The model under review builds one solid part; all positions refer to its coordinate system, in mm. Coordinates: 2 decimals unless noted, no trailing zeros. Write each loop counter-clockwise with the first axis right and the second up, starting at its lowest first coordinate (ties: lowest second). Pieces come first, ordered by that corner, then holes.
1) For line 1 (Y direction, x = 83, z = 0.85); line 2 (X direction, y = 2.5, z = 0.4); line 3 (Y direction, x = -20, z = 0.55), list the stretches that pass through material, from the lowest coordinate up.
2) Add section A-A, the plane x = 0. State the section outline as (y, z) points.
3) Add section C-C, the plane z = 1.5. Give the number of separate pieces and of enclosed holes in the cut face, then the cut area to 3 significant figures.
4) Add section B-B, the plane x = -83. State the section outline as (y, z) points, then the cut area to 3 significant figures.
from build123d import *

# Parameters (mm, degrees)
SKETCH_1_W          = 178
SKETCH_1_H          = 65
EXTRUDE_1_DEPTH     = 3
FILLET_1_R          = 3
SKETCH_2_R          = 2.1
SKETCH_2_R_2        = 12.5
SKETCH_2_R_3        = 11
SKETCH_2_R_4        = 1.8
CUT_EXTRUDE_1_DEPTH = 10


with BuildPart() as part:
    # 草图1 → 凸台-拉伸1 (new body)
    with BuildSketch(Plane.XY):
        Rectangle(SKETCH_1_W, SKETCH_1_H)
    extrude(amount=EXTRUDE_1_DEPTH)

    # 圆角1
    fillet_1_edges = [part.edges().sort_by_distance(p)[0] for p in [
        (-89, 32.5, 1.5),
        (89, 32.5, 1.5),
        (89, -32.5, 1.5),
        (-89, -32.5, 1.5),
    ]]
    fillet(fillet_1_edges, radius=FILLET_1_R)

    # 草图2 → 切除-拉伸1 (cut)
    # profile 1 of 14: a face of its own
    with BuildSketch(Plane.XY.offset(3)):
        with Locations((-83, 27)):
            Circle(SKETCH_2_R)
    # profile 2 of 14: a face of its own
    with BuildSketch(Plane.XY.offset(3)):
        with Locations((-83, 0)):
            Circle(SKETCH_2_R)
    # profile 3 of 14: a face of its own
    with BuildSketch(Plane.XY.offset(3)):
        with Locations((-83, -27)):
            Circle(SKETCH_2_R)
    # profile 4 of 14: a face of its own
    with BuildSketch(Plane.XY.offset(3)):
        Circle(SKETCH_2_R_2)
        Circle(SKETCH_2_R_3, mode=Mode.SUBTRACT)
    # profile 5 of 14: a face of its own
    with BuildSketch(Plane.XY.offset(3)):
        Circle(SKETCH_2_R_3)
    # profile 6 of 14: a face of its own
    with BuildSketch(Plane.XY.offset(3)):
        with Locations((-16.280586137, 23.998802367)):
            Circle(SKETCH_2_R)
        with Locations((-16.280586137, 23.998802367)):
            Circle(SKETCH_2_R_4, mode=Mode.SUBTRACT)
    # profile 7 of 14: a face of its own
    with BuildSketch(Plane.XY.offset(3)):
        with Locations((-16.280586137, 23.998802367)):
            Circle(SKETCH_2_R_4)
    # profile 8 of 14: a face of its own
    with BuildSketch(Plane.XY.offset(3)):
        with Locations((28.923865578, 2.1)):
            Circle(SKETCH_2_R)
        with Locations((28.923865578, 2.1)):
            Circle(SKETCH_2_R_4, mode=Mode.SUBTRACT)
    # profile 9 of 14: a face of its own
    with BuildSketch(Plane.XY.offset(3)):
        with Locations((28.923865578, 2.1)):
            Circle(SKETCH_2_R_4)
    # profile 10 of 14: a face of its own
    with BuildSketch(Plane.XY.offset(3)):
        with Locations((-12.643279441, -26.098802367)):
            Circle(SKETCH_2_R)
    # profile 11 of 14: a face of its own
    with BuildSketch(Plane.XY.offset(3)):
        with BuildLine():
            Line((-15.969193875, -3.766277604), (-16.345745599, 1.420070707))
            ThreePointArc((-16.345745599, 1.420070707), (-16.372108992, 1.547906767), (-16.430660482, 1.664563571))
            ThreePointArc((-16.430660482, 1.664563571), (-16.62644536, 1.833843162), (-16.880639833, 1.882551148))
            Line((-16.880639833, 1.882551148), (-20.471188664, 1.621861493))
            ThreePointArc((-20.471188664, 1.621861493), (-20.813209107, 1.450197211), (-20.933669105, 1.086967259))
            Line((-20.933669105, 1.086967259), (-20.55711738, -4.099381052))
            ThreePointArc((-20.55711738, -4.099381052), (-20.385453099, -4.441401495), (-20.022223146, -4.561861493))
            Line((-20.022223146, -4.561861493), (-16.431674316, -4.301171838))
            ThreePointArc((-16.431674316, -4.301171838), (-16.089653872, -4.129507556), (-15.969193875, -3.766277604))
        make_face()
    # profile 12 of 14: a face of its own
    with BuildSketch(Plane.XY.offset(3)):
        with Locations((83, 27)):
            Circle(SKETCH_2_R)
    # profile 13 of 14: a face of its own
    with BuildSketch(Plane.XY.offset(3)):
        with Locations((83, 0)):
            Circle(SKETCH_2_R)
    # profile 14 of 14: a face of its own
    with BuildSketch(Plane.XY.offset(3)):
        with Locations((83, -27)):
            Circle(SKETCH_2_R)
    extrude(amount=-CUT_EXTRUDE_1_DEPTH, mode=Mode.SUBTRACT)


solid = part.part
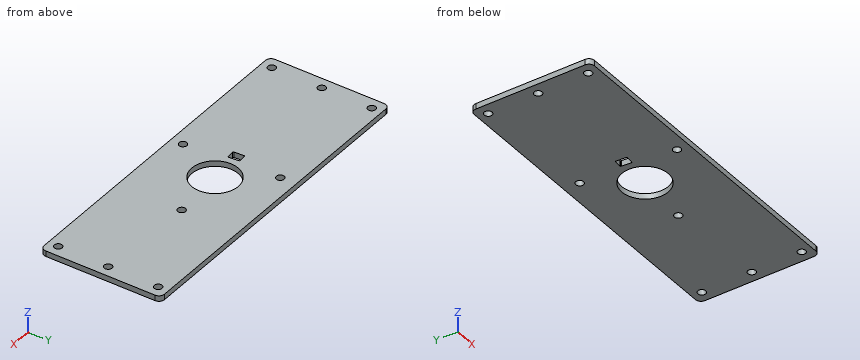
Geometry results:
1. line 1: y = -32.5 to -29.1, -24.9 to -2.1, 2.1 to 24.9, 29.1 to 32.5
1. line 2: x = -89 to -12.25, 12.25 to 26.86, 30.99 to 89
1. line 3: y = -32.5 to -4.56, 1.66 to 32.5
2. outline: (-32.5, 0) - (-12.5, 0) - (-12.5, 3) - (-32.5, 3) - close; (12.5, 0) - (32.5, 0) - (32.5, 3) - (12.5, 3) - close
3. separate pieces: 1
3. enclosed holes: 11
3. area: 10,900 mm2
4. outline: (-32.5, 0) - (-29.1, 0) - (-29.1, 3) - (-32.5, 3) - close; (-24.9, 0) - (-2.1, 0) - (-2.1, 3) - (-24.9, 3) - close; (2.1, 0) - (24.9, 0) - (24.9, 3) - (2.1, 3) - close; (29.1, 0) - (32.5, 0) - (32.5, 3) - (29.1, 3) - close
4. area: 157 mm2
